Source: CAD feature listing. Evaluate the final solid. Frame: model axes, mm. A direction names the side the tool comes from. Give positions to 0.01 mm unless a question says otherwise; leave off trailing zeros. Loops run counter-clockwise (first coordinate to the right, second up) from the corner with the lowest first, then second, coordinate; pieces in that order, holes last. Notation, with made-up numbers: (64.5, 57.5) - (77.5, 57.5) arc R13 cw to (77.5, 82.5) - close; hole circle Ø9 at (-30, 14). An arc over 180 degrees is marked (long way). Put each result on its own line as item: value.
Autodesk Inventor part; units mm, degrees
ref_plane "YZ Plane" through (0, 0, 0) normal (1, 0, 0) x (0, 1, 0)
ref_plane "XZ Plane" through (0, 0, 0) normal (0, 1, 0) x (-1, 0, 0)
ref_plane "XY Plane" through (0, 0, 0) normal (0, 0, 1) x (1, 0, 0)
sketch "Sketch1" plane through (0, 0, 0) normal (0, 1, 0) x (-1, 0, 0)
  circle A0 centre (0, 0) radius 24.13
  circle A1 centre (0, 0) radius 25.4
  line L0 (25.4, 0) -> (0, 0)
  line L1 (0, 0) -> (0, -25.4)
  point P0 (0, -24.13)
  point P1 (24.13, 0)
  dimension "d0" = 48.26
  dimension "d1" = 50.8
extrude "Extrusion1" add sketch "Sketch1" along normal blind 15.24 contours L0 A1 L1 A0 picked at (24.5627, -3.6738)
sketch "Sketch2" plane through (0, 15.24, 0) normal (0, 1, 0) x (1, 0, 0)
  line L0 (-25.0549, 10.8661) -> (-10.8661, 25.0549)
  arc A0 (0, 25.4) -> (-25.4, 0) centre (0, 0) ccw
  line L1 (0, 0) -> (-17.9605, 17.9605)
  line L2 (-25.0549, 10.8661) -> (-23.5944, 9.4056)
  line L3 (-10.8661, 25.0549) -> (-9.4056, 23.5944)
  point P0 (-17.9605, 17.9605)
  dimension "d4" = 20.066
extrude "Extrusion2" add sketch "Sketch2" against normal up to surface (15.24 mm away)
sketch "Sketch3" plane through (0, 15.24, 0) normal (0, 1, 0) x (1, 0, 0)
  line L0 (-24.6957, 11.2253) -> (-11.2253, 24.6957)
  line L1 (-17.9605, 17.9605) -> (-8.9803, 26.9408)
  line L2 (-8.9803, 26.9408) -> (-5.2605, 23.221)
  line L3 (-5.2605, 23.221) -> (-23.221, 5.2605)
  line L4 (-23.221, 5.2605) -> (-26.9408, 8.9803)
  line L5 (-26.9408, 8.9803) -> (-17.9605, 17.9605)
  line L6 (-10.8661, 25.0549) -> (-25.0549, 10.8661)
  line L7 (-5.2605, 23.221) -> (3.175, 20.6375)
  line L8 (3.175, 20.6375) -> (3.175, 30.7046)
  line L9 (3.175, 30.7046) -> (-8.9803, 26.9408)
  line L10 (-26.9408, 8.9803) -> (-30.2776, -1.7961)
  line L11 (-30.2776, -1.7961) -> (-21.5572, -1.7961)
  line L12 (-21.5572, -1.7961) -> (-23.221, 5.2605)
  point P0 (0, 0)
  dimension "d7" = 12.7
  dimension "d8" = 12.7
extrude "Extrusion3" cut sketch "Sketch3" against normal through all contours L4 L12 L11 L10 | L9 L8 L7 L2
properties part number "buttonholderscooterpart"
1) Material intervals for line 1 along Z through (x, y) = (-11.5, 3); line 2 along Z through (x, y) = (-22.25, 12.75); line 3 along X through (y, z) = (12.25, -12.5), sorted ascending. Write a range as [from, to].
Check result:
line 1: [-24.42, -21.21]
line 2: [-13.67, -9.34]
line 3: [-23.42, -20.64]
2) Section query D-D, the plane z = -18.75. Output: boundary loops of the cut face in (x, y).
Check result:
outline: (-17.17, 0) - (-15.19, 0) - (-15.19, 15.24) - (-17.17, 15.24) - close
3) Pin query (flat end, axial travel): P1, Ø6, axis at y = 4.5, z = -20, coming from the -X side; P2, Ø2, axis at x = -22, y = 10, coming from the -Z side; P3, Ø4, axis at x = -12.5, y = 7.5, coming from the +Z side. Return the tip coordinate at first contact, or that it passes through.
Check result:
P1: x = -18.92
P2: z = -14.92
P3: z = -19.29
4) Section query B-B, the plane y = 9.75. Output: boundary loops of the cut face in (x, z), plus the area to 3 significant figures.
Check result:
outline: (-25.05, -10.87) - (-10.87, -25.05) - (-9.41, -23.59) arc R25.4 ccw to (-6.57, -24.53) - (-5.53, -23.49) arc R24.13 cw to (-23.49, -5.53) - (-24.53, -6.57) arc R25.4 ccw to (-23.59, -9.41) - close
area: 47.5 mm²
5) Section query C-C, the plane x = -8.75. Output: boundary loops of the cut face in (y, z).
Check result:
outline: (0, -23.85) - (15.24, -23.85) - (15.24, -22.49) - (0, -22.49) - close
6) Mould query, pull axis Z, two halves, no side actions, for faces 3 (the flat face through (-24, 7.73, -6.04)), 4 (the cylindrical face through (-8.02, 7.51, -24.1)), 5 (the flat face through (-24.335, 7.727, -10.146)), 6 (the cylindrical face through (-24.113, 7.513, -7.984)). Classes: pulls with the +Z half, pulls with the -Z half, needs draft (parallel to the pull), parting line crosses it, or undercut.
Check result:
face 3: pulls with the +Z half
face 4: pulls with the -Z half
face 5: undercut
face 6: undercut
7) Access query for faces 1 (the flat face through (-10.146, 7.727, -24.335)), 2 (the flat face through (-17.4, 15.24, -17.4)). Directions: +Z, -Z, +X, -X, +Y, -Y. A direction counts if a zero-diameter tool reaches every point of the face in a straight line with its end or side. Return the directions, or none.
Check result:
face 1: -Z, +Y, -Y
face 2: +Z, -Z, +X, -X, +Y
8) Section query A-A, the plane z = -24. Output: boundary loops of the cut face in (x, y).
Check result:
outline: (-11.92, 0) - (-9.81, 0) - (-9.81, 15.24) - (-11.92, 15.24) - close; (-8.32, 0) - (-6.04, 0) - (-6.04, 15.24) - (-8.32, 15.24) - close
